```python
from build123d import *

# Parameters (mm, degrees)
F0_W     = 10
F0_H     = 6
F0_W_2   = 8.5
F0_H_2   = 1.2
F1_DEPTH = 8
F2_R     = 0.75
F3_DEPTH = 10
F5_R     = 2


with BuildPart() as f1:
    # F0 (on Top) → F1 (new body)
    with BuildSketch(Plane.XY):
        Rectangle(F0_W, F0_H)
        Rectangle(F0_W_2, F0_H_2, mode=Mode.SUBTRACT)
    extrude(amount=F1_DEPTH)


with BuildPart() as f3:
    # F2 (on face) → F3 (new body)
    with BuildSketch(Plane.YZ.offset(5)):
        with BuildLine():
            Line((-3, 4), (-3, 8))
            Line((-3, 8), (-5, 8))
            ThreePointArc((-5, 8), (-6.414214, 7.414214), (-7, 6))
            Line((-7, 6), (-7, 4))
            Line((-7, 4), (-3, 4))
        make_face()
        with Locations((-5, 6)):
            Circle(F2_R, mode=Mode.SUBTRACT)
        Polygon((-3, 0), (-3, 4), (-7, 4), align=None)
        with BuildLine():
            Line((5, 8), (3, 8))
            Line((3, 8), (3, 4))
            Line((3, 4), (7, 4))
            Line((7, 4), (7, 6))
            ThreePointArc((7, 6), (6.414214, 7.414214), (5, 8))
        make_face()
        with Locations((5, 6)):
            Circle(F2_R, mode=Mode.SUBTRACT)
        Polygon((7, 4), (3, 4), (3, 0), align=None)
    extrude(amount=-F3_DEPTH)


with BuildPart() as f1_1:
    add(f1.part)

    # F4: union F3
    add(f3.part)

    # F5
    f5_edges = [f1_1.edges().sort_by_distance(p)[0] for p in [
        (0, 3, 0),
        (0, 7, 4),
        (0, -3, 0),
        (0, -7, 4),
    ]]
    fillet(f5_edges, radius=F5_R)


solid = f1_1.part
```
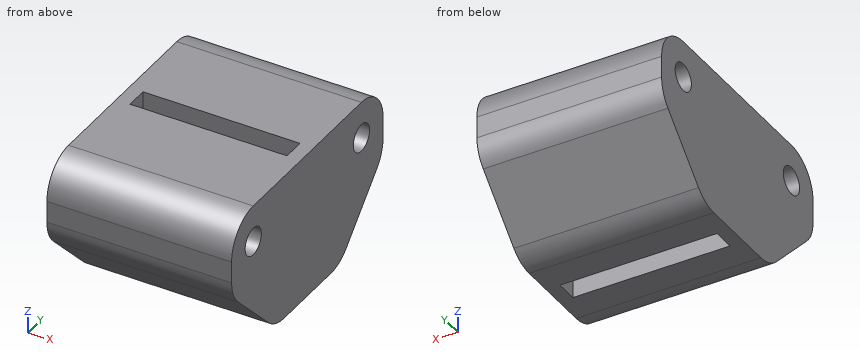
Input: part model. Units: mm. Frame: model coordinates. Round coordinates to 2 decimals unless told otherwise and drop trailing zeros. Order: outer loops, then holes, each group sorted by start corner. A loop starts at its lowest first (then second) coordinate and runs counter-clockwise, first axis right, second up. Notation, with made-up numbers: (5.25, -20.5) - (16.25, -20.5) arc R30 cw to (16.25, 16.5) - close; hole circle Ø9 at (-13, 41.5). An arc over 180 degrees is marked (long way). One line per question, with ' | ' between items. Start each with the question number.
1) Contact query for flat-ended pins moving along their axis: P1, Ø2.5, axis at x = -0.5, z = 2, coming from the +Y side; P2, Ø1.7, axis at y = -5, z = 6, coming from the +X side; P3, Ø2, axis at x = 0, z = 3, coming from the +Y side. Output: stop coordinate, or through.
2) Cut plane A-A, the plane x = 2.5. Return the cut outline in (y, z).
3) Ray query, probe 1 along X at (y, z) = (-0.25, 1.75); probe 2 along Z at (x, y) = (-1.25, -4.5); probe 3 along Y at (x, z) = (0.5, 0.75). Return the intervals inside material, ascending.
4) Cut plane C-C, the plane z = 2. Return the cut outline in (x, y), then the cut area to 3 significant figures.
5) Cut plane B-B, the plane z = 5. Return the cut outline in (x, y).
6) Cut plane D-D, the plane y = 4. Return the cut outline in (x, z), then the cut area to 3 significant figures.
Worked out:
1) P1: stops at y = 6.25 | P2: stops at x = 5 | P3: stops at y = 6.82
2) outline: (-7, 4.83) arc R2 ccw to (-6.41, 3.41) - (-3.59, 0.59) arc R2 ccw to (-2.17, 0) - (-0.6, 0) - (-0.6, 8) - (-5, 8) arc R2 ccw to (-7, 6) - close; (0.6, 0) - (2.17, 0) arc R2 ccw to (3.59, 0.59) - (6.41, 3.41) arc R2 ccw to (7, 4.83) - (7, 6) arc R2 ccw to (5, 8) - (0.6, 8) - close; hole circle Ø1.5 at (-5, 6); hole circle Ø1.5 at (5, 6)
3) probe 1: x = -5 to -4.25, 4.25 to 5 | probe 2: z = 1.5 to 5.44, 6.56 to 8 | probe 3: y = -3.75 to -0.6, 0.6 to 3.75
4) outline: (-5, -5) - (5, -5) - (5, 5) - (-5, 5) - close; hole (-4.25, -0.6) - (4.25, -0.6) - (4.25, 0.6) - (-4.25, 0.6) - close | area: 89.8 mm^2
5) outline: (-5, -7) - (5, -7) - (5, 7) - (-5, 7) - close; hole (-4.25, -0.6) - (4.25, -0.6) - (4.25, 0.6) - (-4.25, 0.6) - close
6) outline: (-5, 1) - (5, 1) - (5, 8) - (-5, 8) - close | area: 70.0 mm^2
